Could you check a few things on this model? Use its own coordinates, in mm. Face numbers are marked on the shaded views. A direction names the side the tool comes from. Round coordinates to 2 decimals unless told otherwise and drop trailing zeros. Loops run counter-clockwise (first coordinate to the right, second up) from the corner with the lowest first, then second, coordinate; pieces in that order, holes last. Notation, with made-up numbers: (-28, 5.5) - (8, 5.5) arc R15 ccw to (8, 32.5) - close; hole circle Ø3 at (-12, -13). An arc over 180 degrees is marked (long way). Use one line per item in the form item = value.
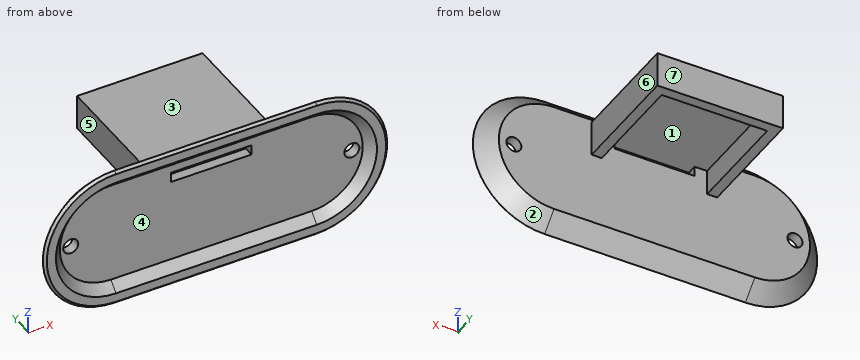
```python
from build123d import *
from OCP.BRepFilletAPI import BRepFilletAPI_MakeChamfer

# Parameters (mm, degrees)
BOSS_EXTRU_1_DEPTH      = 3.8
BOSS_EXTRU_1_TAPER      = 45
COQUE2_DEPTH            = 1.8
COQUE2_DRAFT            = 45
CHANFREIN1_SIZE         = 1
CHANFREIN1_SIZE2        = 0.707106781
ENL_V_MAT_EXTRU_1_REACH = 39.355
ESQUISSE2_R             = 1.5
BOSS_EXTRU_2_DEPTH      = 21
ESQUISSE5_W             = 25
ESQUISSE5_H             = 7
BOSS_EXTRU_3_DEPTH      = 2
ESQUISSE6_W             = 16
ESQUISSE6_H             = 2
ENL_V_MAT_EXTRU_2_DEPTH = 2


# Read off the part's stored shape, not the designer's step: Coque2
with BuildPart() as part:
    # Esquisse1 → Boss.-Extru.1 (new body)
    with BuildSketch(Plane(origin=(0, 0, 0), x_dir=(1, 0, 0), z_dir=(0, 1, 0))):
        with BuildLine():
            ThreePointArc((-20, 14.8), (-34.8, 0), (-20, -14.8))
            Line((-20, -14.8), (20, -14.8))
            ThreePointArc((20, -14.8), (34.8, 0), (20, 14.8))
            Line((20, 14.8), (-20, 14.8))
        make_face()
    extrude(amount=BOSS_EXTRU_1_DEPTH, taper=BOSS_EXTRU_1_TAPER)


with BuildPart() as coque2_tool:
    # Coque2 outline → Coque2 (with draft: the straight prism first)
    with BuildSketch(Plane(origin=(0, 1.8, 0), x_dir=(1, 0, 0), z_dir=(0, 1, 0))):
        with BuildLine():
            Line((-20, -10.171572875), (20, -10.171572875))
            ThreePointArc((20, -10.171572875), (30.171572875, 0), (20, 10.171572875))
            Line((20, 10.171572875), (-20, 10.171572875))
            ThreePointArc((-20, 10.171572875), (-30.171572875, 0), (-20, -10.171572875))
        make_face()
    extrude(amount=-COQUE2_DEPTH)
    # Coque2: the draft: its side faces are tilted about the plane it starts from
    coque2_sides = [coque2_tool.faces().sort_by_distance(p)[0] for p in [
        (0, 0.9, 10.171572875),
        (30.171572875, 0.9, 0),
        (0, 0.9, -10.171572875),
        (-30.171572875, 0.9, 0),
    ]]
    draft(coque2_sides, Plane(origin=(0, 1.8, 0), x_dir=(1, 0, 0), z_dir=(0, 1, 0)), COQUE2_DRAFT)


with BuildPart() as part_1:
    add(part.part)

    # Coque2: cut by coque2_tool
    add(coque2_tool.part, mode=Mode.SUBTRACT)

    # Chanfrein1: one chamfer whose edges measure the first distance from different faces: ONE call of the kernel's chamfer builder (chamfer() names one face for all edges)
    chanfrein1_edges_1 = [part_1.edges().sort_by_distance(p)[0] for p in [
        (0, 0, -14.8),
        (0, 0, 14.8),
        (-34.8, 0, 0),
    ]]
    chanfrein1_side_1 = [part_1.faces().sort_by_distance(p)[0] for p in [
        (0, 0, -14.043672029),
    ]]
    chanfrein1_edges_2 = [part_1.edges().sort_by_distance(p)[0] for p in [
        (34.8, 0, 0),
    ]]
    chanfrein1_side_2 = [part_1.faces().sort_by_distance(p)[0] for p in [
        (32.9, 1.9, 0),
    ]]
    chanfrein1 = BRepFilletAPI_MakeChamfer(part_1.part.solid().wrapped)
    for e in chanfrein1_edges_1:
        chanfrein1.Add(CHANFREIN1_SIZE, CHANFREIN1_SIZE2, e.wrapped, chanfrein1_side_1[0].wrapped)  # the first distance lies on this face
    for e in chanfrein1_edges_2:
        chanfrein1.Add(CHANFREIN1_SIZE, CHANFREIN1_SIZE2, e.wrapped, chanfrein1_side_2[0].wrapped)  # the first distance lies on this face
    add(Compound.cast(chanfrein1.Shape()), mode=Mode.REPLACE)

    # Esquisse2 → Enlèv. mat.-Extru.1 (cut, up to next)
    with BuildSketch(Plane(origin=(0, 3.8, 0), x_dir=(1, 0, 0), z_dir=(0, 1, 0)), mode=Mode.PRIVATE) as enl_v_mat_extru_1_sk1:
        with Locations(Location((-28, 0, 0), (0, 0, 270))):
            Circle(ESQUISSE2_R)
    enl_v_mat_extru_1_tool1 = extrude(enl_v_mat_extru_1_sk1.sketch, amount=-ENL_V_MAT_EXTRU_1_REACH, mode=Mode.PRIVATE) & part_1.part
    # Esquisse2 → Enlèv. mat.-Extru.1 (cut, up to next)
    with BuildSketch(Plane(origin=(0, 3.8, 0), x_dir=(1, 0, 0), z_dir=(0, 1, 0)), mode=Mode.PRIVATE) as enl_v_mat_extru_1_sk2:
        with Locations(Location((28, 0, 0), (0, 0, 270))):
            Circle(ESQUISSE2_R)
    enl_v_mat_extru_1_tool2 = extrude(enl_v_mat_extru_1_sk2.sketch, amount=-ENL_V_MAT_EXTRU_1_REACH, mode=Mode.PRIVATE) & part_1.part
    add(enl_v_mat_extru_1_tool1.solids().sort_by_distance((-28, 3.8, 0))[0], mode=Mode.SUBTRACT)
    add(enl_v_mat_extru_1_tool2.solids().sort_by_distance((28, 3.8, 0))[0], mode=Mode.SUBTRACT)

    # Esquisse3 → Boss.-Extru.2 (add)
    with BuildSketch(Plane(origin=(0, 3.8, 0), x_dir=(1, 0, 0), z_dir=(0, 1, 0))):
        Polygon((-10.5, -8.5), (10.5, -8.5), (10.5, -3.5), (12.5, -3.5), (12.5, -10.5), (-12.5, -10.5), (-12.5, -3.5), (-10.5, -3.5), align=None)
    extrude(amount=BOSS_EXTRU_2_DEPTH)

    # Esquisse5 → Boss.-Extru.3 (add)
    with BuildSketch(Plane(origin=(0, 24.8, 0), x_dir=(1, 0, 0), z_dir=(0, 1, 0))):
        with Locations((0, -7)):
            Rectangle(ESQUISSE5_W, ESQUISSE5_H)
    extrude(amount=BOSS_EXTRU_3_DEPTH)

    # Esquisse6 → Enlèv. mat.-Extru.2 (cut)
    with BuildSketch(Plane(origin=(0, 3.8, 0), x_dir=(1, 0, 0), z_dir=(0, 1, 0))):
        with Locations((0, -7.5)):
            Rectangle(ESQUISSE6_W, ESQUISSE6_H)
    extrude(amount=-ENL_V_MAT_EXTRU_2_DEPTH, mode=Mode.SUBTRACT)


solid = part_1.part
```
1. If we section it at A-A, the plane z = 0: Write out the boundary of the cut face in (x, y).
Solution:
outline = (-34.3, 0.5) - (-33.8, 0) - (-31.97, 0) - (-30.17, 1.8) - (-29.5, 1.8) - (-29.5, 3.8) - (-31, 3.8) - close; (-26.5, 1.8) - (26.5, 1.8) - (26.5, 3.8) - (-26.5, 3.8) - close; (29.5, 1.8) - (30.17, 1.8) - (31.97, 0) - (33.8, 0) - (34.3, 0.5) - (31, 3.8) - (29.5, 3.8) - close
2. If we section it at B-B, the plane y = 21.75: Write out the boundary of the cut face in (x, z).
Solution:
outline = (-12.5, 3.5) - (-10.5, 3.5) - (-10.5, 8.5) - (10.5, 8.5) - (10.5, 3.5) - (12.5, 3.5) - (12.5, 10.5) - (-12.5, 10.5) - close
3. On a 3-axis mill with a long thin cutter (end or side, diameter ignored), from which of +Z, -Z, +X, -X, +Y, -Y can I reach the whole of each face in a straight line? I mean the marked faces 5, 6 and 7. Say none if no direction works.
Solution:
face_5 = +Z, -Z, -X, +Y
face_6 = +Z, -Z, +X, +Y
face_7 = +Z, -Z, +X, -X, +Y
4. We'd pull the mould along X, two halves only. Please class the marked faces 1, 2, 3 and 4: +X half, -X half, draft (parallel to the pull), parting line (faces both ways), or undercut.
Solution:
face_1 = undercut
face_2 = +X half
face_3 = draft
face_4 = undercut
5. Please list where these lines run through material, in increasing order: line 1 along X through (y, z) = (3.2, 0); line 2 along X through (y, z) = (2.6, 0); line 3 along Y through (x, z) = (5, 2).
Solution:
line_1 = -31.6 to -29.5, -26.5 to 26.5, 29.5 to 31.6
line_2 = -32.2 to -29.5, -26.5 to 26.5, 29.5 to 32.2
line_3 = 1.8 to 3.8
6. For P1, Ø1, axis at y = 4.5, z = -8, coming from the -X side; P2, Ø3.5, axis at y = 11.5, z = 8, coming from the +X side; P3, Ø2, axis at x = 2.5, y = 2.5, coming from the +Z side; P4, Ø0.6, axis at y = 3, z = 7.5, coming from the +X side, each with a flat end and sliding along its axis, tell me the tip position at first contact or that it passes through.
Solution:
P1 = through
P2 = 12.5
P3 = 13.3
P4 = 29.56
